Answer from the drawing. Dimensions are ordinates in mm from the lowest x, y and z of the part. Give positions to 0.01 mm unless a question says otherwise; leave off trailing zeros. Order: outer loops, then holes, each group sorted by start corner. A loop starts at its lowest first (then second) coordinate and runs counter-clockwise, first axis right, second up. Notation, with made-up numbers: (76.5, 55.5) - (131.5, 55.5) arc R37 cw to (131.5, 92.5) - close; hole circle Ø8 at (17, 2). An arc over 180 degrees is marked (long way). Answer in a Markdown table with one row per item.
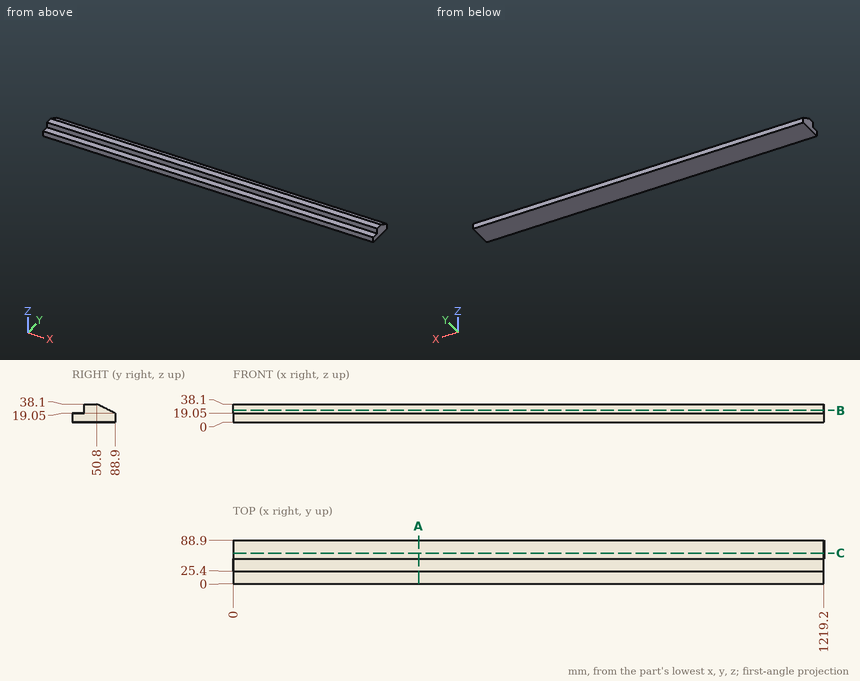
Item 1: Find section A-A on x = 383. Write down the section's boundary in (y, z).
Answer block:
| item | result |
|---|---|
| outline | (0, 0) - (88.9, 0) - (88.9, 19.05) - (50.8, 38.1) - (25.4, 38.1) - (25.4, 19.05) - (0, 19.05) - close |
Item 2: Consider line 1 (Z direction, x = 1003.5, y = 9); line 2 (Z direction, x = 241, y = 53); line 3 (Y direction, x = 785, z = 21). Determine where each line is inside the solid, lowest interval first.
Answer block:
| item | result |
|---|---|
| line 1 | 0 to 19.05 |
| line 2 | 0 to 37 |
| line 3 | 25.4 to 85 |
Item 3: Find section C-C on y = 63. Write down the section's boundary in (x, z).
Answer block:
| item | result |
|---|---|
| outline | (0, 0) - (1219.2, 0) - (1219.2, 32) - (0, 32) - close |
Item 4: Each of these flat-tipped pins is pushed along its axis until it touches: P1, Ø15, axis at x = 719.5, z = 31.5, coming from the -Y side; P2, Ø4, axis at x = 774, z = 28.5, coming from the +Y side; P3, Ø20.5, axis at x = 778.5, y = 7.5, coming from the +Z side. Where does it stop, or does it pass through?
Answer block:
| item | result |
|---|---|
| P1 | y = 25.4 |
| P2 | y = 74 |
| P3 | z = 19.05 |
Item 5: Find section B-B on z = 25. Write down the section's boundary in (x, y), then the cut area to 3 significant figures.
Answer block:
| item | result |
|---|---|
| outline | (0, 25.4) - (1219.2, 25.4) - (1219.2, 77) - (0, 77) - close |
| area | 62,900 mm² |
